from build123d import *

# Parameters (mm, degrees)
BOSS_EXTRUDE1_DEPTH                 = 1.5
F_6_2_6_2_DIAMETER_HOLE1_AT_2_COUNT = 2
F_6_2_6_2_DIAMETER_HOLE1_AT_2_PITCH = 90


with BuildPart() as part:
    # Sketch1 → Boss-Extrude1 (new, symmetric)
    with BuildSketch(Plane(origin=(0, 0, 0), x_dir=(1, 0, 0), z_dir=(0, 1, 0))):
        Polygon((54, 15), (49.5, 15), (49.5, 12), (40.5, 12), (40.5, 15), (31.5, 15), (31.5, 12), (22.5, 12), (22.5, 15), (13.5, 15), (13.5, 12), (4.5, 12), (4.5, 15), (-4.5, 15), (-4.5, 12), (-13.5, 12), (-13.5, 15), (-22.5, 15), (-22.5, 12), (-31.5, 12), (-31.5, 15), (-40.5, 15), (-40.5, 12), (-49.5, 12), (-49.5, 15), (-54, 15), (-54, 12), (-54, 4.5), (-57, 4.5), (-57, -4.5), (-54, -4.5), (-54, -12), (-54, -15), (-49.5, -15), (-49.5, -12), (-40.5, -12), (-40.5, -15), (-31.5, -15), (-31.5, -12), (-22.5, -12), (-22.5, -15), (-13.5, -15), (-13.5, -12), (-4.5, -12), (-4.5, -15), (4.5, -15), (4.5, -12), (13.5, -12), (13.5, -15), (22.5, -15), (22.5, -12), (31.5, -12), (31.5, -15), (40.5, -15), (40.5, -12), (49.5, -12), (49.5, -15), (54, -15), (54, -12), (54, -4.5), (57, -4.5), (57, 4.5), (54, 4.5), (54, 12), align=None)
    extrude(amount=BOSS_EXTRUDE1_DEPTH, both=True)

    # Sketch4 → Ø6.2 (6.2) Diameter Hole1 (revolve, cut)
    with BuildSketch(Plane(origin=(-45, 1.5, -4.5), x_dir=(0, 0, 1), z_dir=(1, 0, 0))):
        Polygon((0, 0), (0, 3), (3.1, 3), (3.1, 0.025), (3.125, 0), align=None)
    f_6_2_6_2_diameter_hole1 = revolve(axis=Axis((-45, 7.85, -4.5), (0, -1, 0)), mode=Mode.SUBTRACT)

    # Ø6.2 (6.2) Diameter Hole1 at 2: Ø6.2 (6.2) Diameter Hole1 ×2
    with Locations(*[(i * F_6_2_6_2_DIAMETER_HOLE1_AT_2_PITCH, 0, 0) for i in range(1, F_6_2_6_2_DIAMETER_HOLE1_AT_2_COUNT)]):
        add(f_6_2_6_2_diameter_hole1, mode=Mode.SUBTRACT)


solid = part.part
CAD build for the part. Positions are in the model's coordinates, mm. A direction names the side the tool comes from. Coordinates: 2 decimals unless noted, no trailing zeros. Loops run counter-clockwise (first coordinate to the right, second up) from the corner with the lowest first, then second, coordinate; pieces in that order, holes last. Notation, with made-up numbers: (61, -8) - (92, -8) arc R21 cw to (92, 15) - close; hole circle Ø8 at (29.25, 87). An arc over 180 degrees is marked (long way). Write item = value, one per line. Start each with the question number.
Q1. Cut at A-A, the plane x = 45. List the corners of the cut face in (y, z) (3 decimals).
Q2. Cut at C-C, the plane z = -9. List the corners of the cut face in (x, y), then the cut area to 3 significant figures.
Q3. Flat gauge pins, fed straight in: pin 1 Ø0.9 at (x, y) = (8.5, 0.5) entering from -Z; pin 2 Ø1.5 at (y, z) = (-0.5, -14) entering from -X; pin 3 Ø1.5 at (x, y) = (-55, 0) entering from +Z. Where does each tip first touch, or does it go through?
Q4. Cut at D-D, the plane x = -25.5. List the corners of the cut face in (y, z), then the cut area to 3 significant figures.
Q5. Pull direction X, two halves, no side cores. Call faces 1 (the flat face through (-57, 0, 0)), 2 (the flat face through (22.5, 0, 14)), 3 (the flat face through (-18, 0, -15)): pulls with the +X half, pulls with the -X half, needs draft (parallel to the pull), parting line crosses it, or undercut.
Q6. Which spindle directions (+Z, -Z, +X, -X, +Y, -Y) get a long thin tool onto all of the face, cutting with end or side? Do faces 4 (the flat face through (-4.5, 0, 13)), 5 (the flat face through (52, 0, 15)), 6 (the flat face through (-56, 0, 4.5)), 7 (the cylindrical face through (41.926, 0.008, -4.904)), 8 (the flat face through (13.5, 0, -14)). Say none if no direction does.
Q7. Cut at B-B, the plane y = 0.35. Give the number of separate pieces and of enclosed holes in the cut face, then the cut area to 3 significant figures.
Q8. Drill centre lines: L1, parallel to Z at x = 45, y = 0.35; L2, parallel to X at y = 1.4, z = -2.5; L3, parallel to X at y = 0.5, z = -11. Where is each one in solid material? Low to high.
Computed:
q1.outline = (-1.5, -12) - (1.5, -12) - (1.5, -7.625) - (1.475, -7.6) - (-1.5, -7.6) - close; (-1.5, -1.4) - (1.475, -1.4) - (1.5, -1.375) - (1.5, 12) - (-1.5, 12) - close
q2.outline = (-54, -1.5) - (54, -1.5) - (54, 1.5) - (-54, 1.5) - close
q2.area = 324 mm²
q3.pin_1 = -12
q3.pin_2 = -54
q3.pin_3 = 4.5
q4.outline = (-1.5, -12) - (1.5, -12) - (1.5, 12) - (-1.5, 12) - close
q4.area = 72.0 mm²
q5.face_1 = pulls with the -X half
q5.face_2 = undercut
q5.face_3 = needs draft
q6.face_4 = +Z, +Y, -Y
q6.face_5 = +Z, +X, -X, +Y, -Y
q6.face_6 = +Z, -X, +Y, -Y
q6.face_7 = +Y, -Y
q6.face_8 = -Z, +Y, -Y
q7.separate_pieces = 1
q7.enclosed_holes = 2
q7.area = 2,910 mm²
q8.L1 = -12 to -7.6, -1.4 to 12
q8.L2 = -57 to -47.37, -42.63 to 42.63, 47.37 to 57
q8.L3 = -54 to 54
